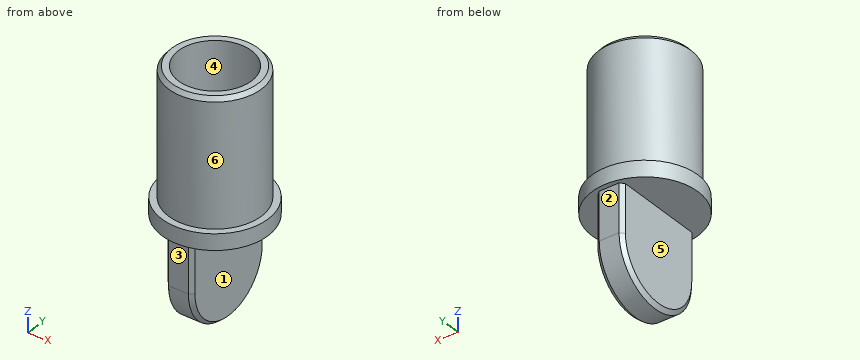
```python
from build123d import *
from OCP.BRepFilletAPI import BRepFilletAPI_MakeChamfer

# Parameters (mm, degrees)
SKETCH1_R           = 7.325878031
EXTRUDE1_DEPTH      = 30.082981268
EXTRUDE4_DEPTH      = 32.817019656
EXTRUDE4_DEPTH_BACK = 32.817019656
SKETCH2_R           = 7.578564767
SKETCH2_5_R         = 7.578564767
EXTRUDE5_DEPTH      = 2.159
SKETCH3_R           = 8.388232563
EXTRUDE6_DEPTH      = 2.54
CHAMFER1_SIZE       = 0.635
CHAMFER1_SIZE2      = 0.532828266
CHAMFER2_SIZE       = 0.635
CHAMFER2_SIZE2      = 0.532828266
SKETCH4_R           = 5.776692344
EXTRUDE7_DEPTH      = 19.964416501


with BuildPart() as part:
    # Sketch1 → Extrude1 (new body)
    with BuildSketch(Plane.XY):
        with Locations(Location((0, 0, 0), (0, 0, 180))):
            Circle(SKETCH1_R)
    extrude(amount=EXTRUDE1_DEPTH)

    # Sketch2 → Extrude4 (cut, two sides: drawn at the far end of the back side and taken through both)
    with BuildSketch(Plane(origin=(0, 0, 0), x_dir=(0, 0, -1), z_dir=(1, 0, 0)).offset(-EXTRUDE4_DEPTH_BACK)):
        Circle(SKETCH2_R)
        with BuildLine():
            ThreePointArc((-7.578564767, 0), (-5.358854538, 5.358854538), (0, 7.578564767))
            Line((0, 7.578564767), (-7.578564767, 7.578564767))
            Line((-7.578564767, 7.578564767), (-7.578564767, 0))
        make_face()
        with BuildLine():
            ThreePointArc((0, -7.578564767), (-5.358854538, -5.358854538), (-7.578564767, 0))
            Line((-7.578564767, 0), (-7.578564767, -7.578564767))
            Line((-7.578564767, -7.578564767), (0, -7.578564767))
        make_face()
    extrude(amount=EXTRUDE4_DEPTH + EXTRUDE4_DEPTH_BACK, mode=Mode.SUBTRACT)

    # Sketch2<5> → Extrude5 (add, symmetric)
    with BuildSketch(Plane(origin=(0, 0, 0), x_dir=(0, 0, -1), z_dir=(1, 0, 0))):
        with BuildLine():
            ThreePointArc((-7.578564767, 0), (-5.358854538, 5.358854538), (0, 7.578564767))
            Line((0, 7.578564767), (-7.578564767, 7.578564767))
            Line((-7.578564767, 7.578564767), (-7.578564767, 0))
        make_face()
        Circle(SKETCH2_5_R)
        with BuildLine():
            ThreePointArc((0, -7.578564767), (-5.358854538, -5.358854538), (-7.578564767, 0))
            Line((-7.578564767, 0), (-7.578564767, -7.578564767))
            Line((-7.578564767, -7.578564767), (0, -7.578564767))
        make_face()
    extrude(amount=EXTRUDE5_DEPTH, both=True)

    # Sketch3 → Extrude6 (add)
    with BuildSketch(Plane(origin=(0, 0, 7.578564767), x_dir=(-1, 0, 0), z_dir=(0, 0, -1))):
        Circle(SKETCH3_R)
    extrude(amount=-EXTRUDE6_DEPTH)

    # Chamfer1: one chamfer whose edges measure the first distance from different faces: ONE call of the kernel's chamfer builder (chamfer() names one face for all edges)
    chamfer1_edges_1 = [part.edges().sort_by_distance(p)[0] for p in [
        (-2.159, -7.578564767, 3.789282384),
        (-2.159, 0, -7.578564767),
        (-2.159, 7.578564767, 3.789282384),
    ]]
    chamfer1_side_1 = [part.faces().sort_by_distance(p)[0] for p in [
        (-2.159, 0, 0.707457952),
    ]]
    chamfer1_edges_2 = [part.edges().sort_by_distance(p)[0] for p in [
        (2.159, -7.578564767, 3.789282384),
    ]]
    chamfer1_side_2 = [part.faces().sort_by_distance(p)[0] for p in [
        (0, -7.578564767, 3.789282384),
    ]]
    chamfer1_edges_3 = [part.edges().sort_by_distance(p)[0] for p in [
        (2.159, 0, -7.578564767),
    ]]
    chamfer1_side_3 = [part.faces().sort_by_distance(p)[0] for p in [
        (0, 0, -7.578564767),
    ]]
    chamfer1_edges_4 = [part.edges().sort_by_distance(p)[0] for p in [
        (2.159, 7.578564767, 3.789282384),
    ]]
    chamfer1_side_4 = [part.faces().sort_by_distance(p)[0] for p in [
        (0, 7.578564767, 3.789282384),
    ]]
    chamfer1 = BRepFilletAPI_MakeChamfer(part.part.solid().wrapped)
    for e in chamfer1_edges_1:
        chamfer1.Add(CHAMFER1_SIZE, CHAMFER1_SIZE2, e.wrapped, chamfer1_side_1[0].wrapped)  # the first distance lies on this face
    for e in chamfer1_edges_2:
        chamfer1.Add(CHAMFER1_SIZE, CHAMFER1_SIZE2, e.wrapped, chamfer1_side_2[0].wrapped)  # the first distance lies on this face
    for e in chamfer1_edges_3:
        chamfer1.Add(CHAMFER1_SIZE, CHAMFER1_SIZE2, e.wrapped, chamfer1_side_3[0].wrapped)  # the first distance lies on this face
    for e in chamfer1_edges_4:
        chamfer1.Add(CHAMFER1_SIZE, CHAMFER1_SIZE2, e.wrapped, chamfer1_side_4[0].wrapped)  # the first distance lies on this face
    add(Compound.cast(chamfer1.Shape()), mode=Mode.REPLACE)

    # Chamfer2
    chamfer2_edges = [part.edges().sort_by_distance(p)[0] for p in [
        (7.325878031, 0, 30.082981268),
    ]]
    chamfer2_side = [part.faces().sort_by_distance(p)[0] for p in [
        (7.325878031, 0, 20.100773018),
    ]]
    chamfer(chamfer2_edges, length=CHAMFER2_SIZE, length2=CHAMFER2_SIZE2, reference=chamfer2_side[0])

    # Sketch4 → Extrude7 (cut)
    with BuildSketch(Plane.XY.offset(30.082981268)):
        Circle(SKETCH4_R)
    extrude(amount=-EXTRUDE7_DEPTH, mode=Mode.SUBTRACT)


solid = part.part
```
Source: CAD feature listing. Evaluate the final solid. Frame: model axes, mm. Face numbers are marked on the shaded views. A direction names the side the tool comes from. Give positions to 0.01 mm unless a question says otherwise; leave off trailing zeros. Loops run counter-clockwise (first coordinate to the right, second up) from the corner with the lowest first, then second, coordinate; pieces in that order, holes last. Notation, with made-up numbers: (-6.5, -3) - (36.5, -3) arc R24 ccw to (36.5, 7) - close; hole circle Ø11 at (59.5, 71). An arc over 180 degrees is marked (long way). Use CSV: the item, a comma, the result in double quotes.
1) Cut plane C-C (z = 2). Output: boundary loops of the cut face in (x, y).
Worked out:
outline,"(-2.16, -6.94) - (-1.63, -7.58) - (1.52, -7.58) - (2.16, -7.05) - (2.16, 7.05) - (1.52, 7.58) - (-1.63, 7.58) - (-2.16, 6.94) - close"
2) Set-up query: the marked faces 1, 2 and 3. Return all of +Z, -Z, +X, -X, +Y, -Y with unobstructed straight access to the full face (end or side cutting, diameter ignored); none if empty.
Worked out:
face 1,"-Z, +X, +Y, -Y"
face 2,"-Z, +X, -X, +Y"
face 3,"-Z, +X, -X, -Y"
3) Cut plane D-D (z = 16). Output: boundary loops of the cut face in (x, y).
Worked out:
outline,"circle Ø14.65 at (0, 0); hole circle Ø11.55 at (0, 0)"
4) Mould query, pull axis Y, two halves, no side actions, for the marked faces 4, 5 and 6. Classes: +Y half, -Y half, draft (parallel to the pull), parting line (faces both ways), or undercut.
Worked out:
face 4,"undercut"
face 5,"draft"
face 6,"parting line"
5) Cut plane A-A (x = 0). Output: boundary loops of the cut face in (y, z).
Worked out:
outline,"(-8.39, 7.58) - (-7.58, 7.58) - (-7.58, 0) arc R7.58 ccw to (7.58, 0) - (7.58, 7.58) - (8.39, 7.58) - (8.39, 10.12) - (7.33, 10.12) - (7.33, 29.45) - (6.79, 30.08) - (5.78, 30.08) - (5.78, 10.12) - (-5.78, 10.12) - (-5.78, 30.08) - (-6.79, 30.08) - (-7.33, 29.45) - (-7.33, 10.12) - (-8.39, 10.12) - close"
6) Line query: line 1 (Y direction, x = 0, z = 20.75); line 2 (Z direction, x = -6, y = 0.25); line 3 (Z direction, x = 2.25, y = -1.25). Output: solid intervals per line, ascending.
Worked out:
line 1,"y = -7.33 to -5.78, 5.78 to 7.33"
line 2,"z = 7.58 to 30.08"
line 3,"z = 7.58 to 10.12"
7) Cut plane B-B (y = 0). Output: boundary loops of the cut face in (x, z), and give its area (3 significant figures).
Worked out:
outline,"(-8.39, 7.58) - (-2.16, 7.58) - (-2.16, -6.94) - (-1.63, -7.58) - (1.52, -7.58) - (2.16, -7.05) - (2.16, 7.58) - (8.39, 7.58) - (8.39, 10.12) - (7.33, 10.12) - (7.33, 29.45) - (6.79, 30.08) - (5.78, 30.08) - (5.78, 10.12) - (-5.78, 10.12) - (-5.78, 30.08) - (-6.79, 30.08) - (-7.33, 29.45) - (-7.33, 10.12) - (-8.39, 10.12) - close"
area,"169 mm^2"
8) Pin query (flat end, axial travel): P1, Ø1.6, axis at x = 0.5, z = 4.5, coming from the +Y side; P2, Ø5, axis at x = -3.5, y = 3, coming from the -Z side; P3, Ø3, axis at x = -3.5, z = 10, coming from the +Y side; P4, Ø6, axis at x = -3, z = 10.5, coming from the -Y side. Return the tip coordinate at first contact, or that it passes through.
Worked out:
P1,"stops at y = 7.58"
P2,"stops at z = -7.46"
P3,"stops at y = 8.15"
P4,"stops at y = -8.39"
